```python
from build123d import *
from build123d.topology import SkipClean

# Parameters (mm, degrees)
EXTRUDE_1_DEPTH   = 10
EXTRUDE_1_2_DEPTH = 10
SKETCH_4_R        = 5
EXTRUDE_3_DEPTH   = 12
SKETCH_7_R        = 5
EXTRUDE_4_DEPTH   = 12


with BuildPart() as part:
    # 草图1 → Extrude 1 (new body)
    with BuildSketch(Plane.XY):
        with BuildLine():
            Line((50, 0), (50, 49))
            ThreePointArc((50, 49), (45.606601718, 59.606601718), (35, 64))
            Line((35, 64), (-35, 64))
            ThreePointArc((-35, 64), (-45.606601718, 59.606601718), (-50, 49))
            Line((-50, 49), (-50, 0))
            Line((-50, 0), (-40, 0))
            Line((-40, 0), (-40, 49))
            ThreePointArc((-40, 49), (-38.535533906, 52.535533906), (-35, 54))
            Line((-35, 54), (35, 54))
            ThreePointArc((35, 54), (38.535533906, 52.535533906), (40, 49))
            Line((40, 49), (40, 0))
            Line((40, 0), (50, 0))
        make_face()
    extrude(amount=EXTRUDE_1_DEPTH)

    # 草图2 → Extrude 1 2 (add)
    with BuildSketch(Plane(origin=(50, 0, 0), x_dir=(0, 0, -1), z_dir=(1, 0, 0))):
        with BuildLine():
            Line((0, 17.071067812), (0, 0))
            Line((0, 0), (-18, 0))
            ThreePointArc((-18, 0), (-22.619397663, 3.086582838), (-21.535533906, 8.535533906))
            Line((-21.535533906, 8.535533906), (-10, 20.071067812))
            Line((-10, 20.071067812), (0, 20.071067812))
            Line((0, 20.071067812), (0, 17.071067812))
        make_face()
    extrude_1_2 = extrude(amount=-EXTRUDE_1_2_DEPTH)

    # 草图4 → 凸台-拉伸3 (add)
    with BuildSketch(Plane.ZY.offset(-40)):
        with Locations(Location((18, 5, 0), (0, 0, 270))):
            Circle(SKETCH_4_R)
    extrude_3 = extrude(amount=EXTRUDE_3_DEPTH)

    # 镜向3: Extrude 1 2, 凸台-拉伸3 across plane
    add(extrude_1_2.mirror(Plane(origin=(0, 0, 0), x_dir=(0, 0, 1), z_dir=(1, 0, 0))))
    add(extrude_3.mirror(Plane(origin=(0, 0, 0), x_dir=(0, 0, 1), z_dir=(1, 0, 0))))

    # 草图7 → 凸台-拉伸4 (add)
    with SkipClean():  # the faces are left unmerged after this step: merging them gives an invalid solid
        with BuildSketch(Plane(origin=(50, 0, 0), x_dir=(0, 0, -1), z_dir=(1, 0, 0))):
            with Locations((-18, 5)):
                Circle(SKETCH_7_R)
        extrude_4 = extrude(amount=EXTRUDE_4_DEPTH)

    # 镜向4: 凸台-拉伸4 across plane
    with SkipClean():  # the faces are left unmerged after this step: merging them gives an invalid solid
        add(extrude_4.mirror(Plane(origin=(0, 0, 0), x_dir=(0, 0, 1), z_dir=(1, 0, 0))))


solid = part.part
```
CAD build for the part. Positions are in the model's coordinates, mm. A direction names the side the tool comes from. Round coordinates to 2 decimals unless told otherwise and drop trailing zeros. Order: outer loops, then holes, each group sorted by start corner. A loop starts at its lowest first (then second) coordinate and runs counter-clockwise, first axis right, second up. Notation, with made-up numbers: (81.25, 62) - (129.25, 62) arc R18 ccw to (129.25, 93) - close; hole circle Ø6 at (-39, -10). An arc over 180 degrees is marked (long way). Answer in a Markdown table with one row per item. Add a question column.
(1) Band-saw the part on D-D on y = 5. List the corners of the cut face in (x, z), and give its area (3 significant figures).
(2) Mould opens along X. For faces 4 (the face through (0, 56, 0)), 5 (the face through (-62, 5, 18)), 6 (the face through (40, 25, 6)) say: +X half, -X half, draft (parallel to the pull), parting line (faces both ways), or undercut.
(3) Band-saw the part on B-B on x = -30. List the corners of the cut face in (y, z), and give its area (3 significant figures).
(4) Band-saw the part on A-A on y = 39.5. List the corners of the cut face in (x, z), and give its area (3 significant figures).
(5) Band-saw the part on C-C on z = 19.5. List the corners of the cut face in (x, y), and give its area (3 significant figures).
(6) 3-axis set-ups, long thin cutter, end or side, ignore diameter. For faces 1 (the face through (-28, 5, 18)), 2 (the face through (0, 54, 5)), 3 (the face through (-1, 57, 10)): which of +Z, -Z, +X, -X, +Y, -Y reach the whole face in a straight line?
(7) Drop flat-ended pins along their axis: pin 1 Ø11 at (y, z) = (17.5, 12.5) entering from +X; pin 2 Ø1 at (x, z) = (39, 3) entering from -Y; pin 3 Ø5 at (x, y) = (-16.5, 54.5) entering from +Z. Give the stop position or say it passes through.
(8) Probe L1, parallel to X at y = 28, z = 3.5; L2, parallel to X at y = 9, z = 16; L3, parallel to Y at x = 0, z = 3. List the from-to ranges inside material, lowest first. Write a range as [from, to].
Data:
| question | item | result |
|---|---|---|
| 1 | outline | (-62, 13) - (-50, 13) - (-50, 0) - (-40, 0) - (-40, 13) - (-28, 13) - (-28, 23) - (-62, 23) - close; (28, 13) - (40, 13) - (40, 0) - (50, 0) - (50, 13) - (62, 13) - (62, 23) - (28, 23) - close |
| 1 | area | 940 mm^2 |
| 2 | face 4 | draft |
| 2 | face 5 | -X half |
| 2 | face 6 | undercut |
| 3 | outline | circle Ø10 at (5, 18); (54, 0) - (64, 0) - (64, 10) - (54, 10) - close |
| 3 | area | 179 mm^2 |
| 4 | outline | (-50, 0) - (-40, 0) - (-40, 10) - (-50, 10) - close; (40, 0) - (50, 0) - (50, 10) - (40, 10) - close |
| 4 | area | 200 mm^2 |
| 5 | outline | (-62, 0.23) - (-28, 0.23) - (-28, 9.77) - (-40, 9.77) - (-40, 10.57) - (-50, 10.57) - (-50, 9.77) - (-62, 9.77) - close; (28, 0.23) - (62, 0.23) - (62, 9.77) - (50, 9.77) - (50, 10.57) - (40, 10.57) - (40, 9.77) - (28, 9.77) - close |
| 5 | area | 665 mm^2 |
| 6 | face 1 | +Z, -Z, +Y, -Y |
| 6 | face 2 | +Z, -Z, -Y |
| 6 | face 3 | +Z, +X, -X, +Y |
| 7 | pin 1 | stops at x = 50 |
| 7 | pin 2 | stops at y = 51.18 |
| 7 | pin 3 | stops at z = 10 |
| 8 | L1 | x = [-50, -40], [40, 50] |
| 8 | L2 | x = [-62, -28], [28, 62] |
| 8 | L3 | y = [54, 64] |
